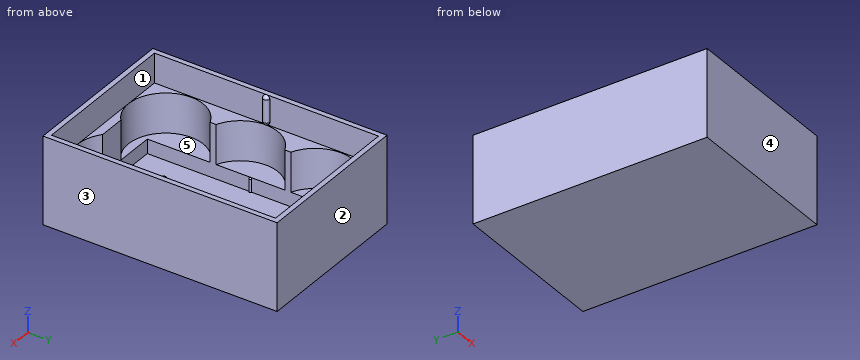
```python
from build123d import *

# Parameters (mm, degrees)
F0_W      = 94
F0_H      = 137.5
F1_DEPTH  = 2.5
F2_W      = 94
F2_H      = 137.5
F2_W_2    = 62
F2_H_2    = 123
F3_DEPTH  = 8.5
F4_W      = 94
F4_H      = 137.5
F5_DEPTH  = 23.5
F6_W      = 62
F6_H      = 123
F7_DEPTH  = 23.501
F8_W      = 94
F8_H      = 137.5
F8_W_2    = 90
F8_H_2    = 133.5
F9_DEPTH  = 17.5
F11_ANGLE = 180
F13_ANGLE = 180
F14_W     = 0.75
F14_H     = 7.75
F16_W     = 0.75
F16_H     = 7.75
F19_DEPTH = 1
F20_DEPTH = 1
F21_DEPTH = 1
F22_DEPTH = 1


with BuildPart() as f1:
    # F0 (on Top) → F1 (new body)
    with BuildSketch(Plane.XY):
        Rectangle(F0_W, F0_H)
    extrude(amount=F1_DEPTH)

    # F2 (on face) → F3 (join)
    with BuildSketch(Plane.XY.offset(2.5)):
        Rectangle(F2_W, F2_H)
        Rectangle(F2_W_2, F2_H_2, mode=Mode.SUBTRACT)
    extrude(amount=F3_DEPTH)

    # F4 (on face) → F5 (join)
    with BuildSketch(Plane.XY.offset(11)):
        Rectangle(F4_W, F4_H)
        with BuildLine():
            ThreePointArc((-22.25, 22.25), (-37.9831258814, 60.2331258814), (0, 44.5))
            ThreePointArc((0, 44.5), (22.25, 66.75), (44.5, 44.5))
            ThreePointArc((44.5, 44.5), (37.9831258872, 28.7668741244), (22.2500000164, 22.25))
            ThreePointArc((22.2500000164, 22.25), (37.9831258872, 15.7331258756), (44.5, 0))
            ThreePointArc((44.5, 0), (37.9831258814, -15.7331258814), (22.25, -22.25))
            ThreePointArc((22.25, -22.25), (37.9831258814, -28.7668741186), (44.5, -44.5))
            ThreePointArc((44.5, -44.5), (22.25, -66.75), (0, -44.5))
            ThreePointArc((0, -44.5), (-37.983125897, -60.2331258658), (-22.249999956, -22.25))
            ThreePointArc((-22.249999956, -22.25), (-44.5, -2.2e-08), (-22.25, 22.25))
        make_face(mode=Mode.SUBTRACT)
    extrude(amount=F5_DEPTH)

    # F6 (on face) → F7 (cut, through all)
    with BuildSketch(Plane.XY.offset(11)):
        Rectangle(F6_W, F6_H)
    extrude(amount=F7_DEPTH, mode=Mode.SUBTRACT)

    # F8 (on face) → F9 (join)
    with BuildSketch(Plane.XY.offset(34.5)):
        Rectangle(F8_W, F8_H)
        Rectangle(F8_W_2, F8_H_2, mode=Mode.SUBTRACT)
    extrude(amount=F9_DEPTH)

    # F10 (on face) → F11 (revolve)
    with BuildSketch(Plane.YZ.offset(-45)):
        with BuildLine():
            Line((0, 36.5), (0, 34.5))
            ThreePointArc((0, 34.5), (1.4142135624, 35.0857864376), (2, 36.5))
            Line((2, 36.5), (2, 50))
            ThreePointArc((2, 50), (1.4142135624, 51.4142135624), (0, 52))
            Line((0, 52), (0, 50))
            Line((0, 50), (0, 36.5))
        make_face()
    revolve(axis=Axis((-45, 0, 43.25), (0, 0, -1)), revolution_arc=F11_ANGLE)

    # F12 (on face) → F13 (revolve)
    with BuildSketch(Plane(origin=(45, 0, 0), x_dir=(0, -1, 0), z_dir=(-1, 0, 0))):
        with BuildLine():
            ThreePointArc((-2, 36.5), (-1.4142135624, 35.0857864376), (0, 34.5))
            Line((0, 34.5), (0, 36.5))
            Line((0, 36.5), (0, 50))
            Line((0, 50), (-2, 50))
            Line((-2, 50), (-2, 36.5))
        make_face()
        with BuildLine():
            Line((-2, 50), (0, 50))
            Line((0, 50), (0, 52))
            ThreePointArc((0, 52), (-1.4142135624, 51.4142135624), (-2, 50))
        make_face()
    revolve(axis=Axis((45, 0, 43.25), (0, 0, 1)), revolution_arc=F13_ANGLE)

    # F14 (on face) → F15 (revolve)
    with BuildSketch(Plane.YZ.offset(-31)):
        with BuildLine():
            ThreePointArc((0.75, 10.25), (0.5303300859, 10.7803300859), (0, 11))
            Line((0, 11), (0, 10.25))
            Line((0, 10.25), (0.75, 10.25))
        make_face()
        with Locations((0.375, 6.375)):
            Rectangle(F14_W, F14_H)
    revolve(axis=Axis((-31, 0, 6.75), (0, 0, -1)))

    # F16 (on face) → F17 (revolve)
    with BuildSketch(Plane(origin=(31, 0, 0), x_dir=(0, -1, 0), z_dir=(-1, 0, 0))):
        with Locations((-0.375, 6.375)):
            Rectangle(F16_W, F16_H)
        with BuildLine():
            Line((-0.75, 10.25), (0, 10.25))
            Line((0, 10.25), (0, 11))
            ThreePointArc((0, 11), (-0.5303300859, 10.7803300859), (-0.75, 10.25))
        make_face()
    revolve(axis=Axis((31, 0, 6.75), (0, 0, 1)))

    # F19 (add): a face of the model
    f19_faces = [f1.faces().sort_by_distance(p)[0] for p in [
        (47, 0, 26),
    ]]
    extrude(f19_faces, amount=F19_DEPTH)

    # F20 (add): a face of the model
    f20_faces = [f1.faces().sort_by_distance(p)[0] for p in [
        (-47, 0, 26),
    ]]
    extrude(f20_faces, amount=F20_DEPTH)

    # F21 (add): a face of the model
    f21_faces = [f1.faces().sort_by_distance(p)[0] for p in [
        (0, -68.75, 26),
    ]]
    extrude(f21_faces, amount=F21_DEPTH)

    # F22 (add): a face of the model
    f22_faces = [f1.faces().sort_by_distance(p)[0] for p in [
        (0, 68.75, 26),
    ]]
    extrude(f22_faces, amount=F22_DEPTH)


solid = f1.part
```
Source: CAD feature listing. Evaluate the final solid. Frame: model axes, mm. Face numbers are marked on the shaded views. A direction names the side the tool comes from. Round coordinates to 2 decimals unless told otherwise and drop trailing zeros. Order: outer loops, then holes, each group sorted by start corner. A loop starts at its lowest first (then second) coordinate and runs counter-clockwise, first axis right, second up. Notation, with made-up numbers: (62, 59.5) -> (108, 59.5) arc R25 cw to (108, 84.5) -> close; hole circle Ø9 at (83, -10). An arc over 180 degrees is marked (long way). One line per item, written item: value. Start each with the question number.
Q1. Access query for the marked faces 4 and 5. Directions: +Z, -Z, +X, -X, +Y, -Y. A direction counts if a zero-diameter tool reaches every point of the face in a straight line with its end or side. Return the directions, or none.
Q2. Section query C-C (x = 24). Return the cut outline in (y, z), plus the area to 3 significant figures.
Q3. Draft query along X for the marked faces 1, 2 and 3. Return one class per face: pulls with the +X half, pulls with the -X half, needs draft (parallel to the pull), parting line crosses it, or undercut.
Q4. Pin query (flat end, axial travel): pin 1 (11 mm diameter, centred on x = 36, y = 0.5, fed in from +Z); pin 2 (7 mm diameter, centred on x = -39.5, y = -10, fed in from +Z). Return the tip coordinate at first contact, or that it passes through.
Q5. Section query A-A (z = 23.5). Return the cut outline in (x, y), plus the area to 3 significant figures.
Q6. Section query D-D (z = 38.5). Return the cut outline in (x, y).
Q7. Section query B-B (y = 44.5). Return the cut outline in (x, z).
Q8. Material intervals for probe 1 along Y at (x, z) = (2, 44); probe 2 along X at (y, z) = (29.5, 36); probe 3 along Y at (x, z) = (35.5, 29.5), sorted ascending.
Findings below:
1. face 4: +Z, -Z, +X, -X, -Y
1. face 5: +Z
2. outline: (-69.75, 0) -> (69.75, 0) -> (69.75, 52) -> (66.75, 52) -> (66.75, 34.5) -> (66.68, 34.5) -> (66.68, 11) -> (61.5, 11) -> (61.5, 2.5) -> (-61.5, 2.5) -> (-61.5, 11) -> (-66.68, 11) -> (-66.68, 34.5) -> (-66.75, 34.5) -> (-66.75, 52) -> (-69.75, 52) -> close
2. area: 738 mm²
3. face 1: undercut
3. face 2: needs draft
3. face 3: pulls with the +X half
4. pin 1: z = 11
4. pin 2: z = 34.5
5. outline: (-48, -69.75) -> (48, -69.75) -> (48, 69.75) -> (-48, 69.75) -> close; hole (-31, -24.04) arc R22.25 ccw (long way) to (-7.9, -61.5) -> (7.9, -61.5) arc R22.25 ccw (long way) to (31, -24.04) -> (31, -20.46) arc R22.25 ccw to (31, 20.46) -> (31, 24.04) arc R22.25 ccw (long way) to (7.9, 61.5) -> (-7.9, 61.5) arc R22.25 ccw (long way) to (-31, 24.04) -> (-31, 20.46) arc R22.25 ccw to (-31, -20.46) -> close
5. area: 3,010 mm²
6. outline: (-48, -69.75) -> (48, -69.75) -> (48, 69.75) -> (-48, 69.75) -> close; hole (-45, -66.75) -> (45, -66.75) -> (45, -2) arc R2 cw to (45, 2) -> (45, 66.75) -> (-45, 66.75) -> (-45, 2) arc R2 cw to (-45, -2) -> close
7. outline: (-48, 0) -> (48, 0) -> (48, 52) -> (45, 52) -> (45, 34.5) -> (44.5, 34.5) -> (44.5, 11) -> (31, 11) -> (31, 2.5) -> (-31, 2.5) -> (-31, 11) -> (-44.5, 11) -> (-44.5, 34.5) -> (-45, 34.5) -> (-45, 52) -> (-48, 52) -> close
8. probe 1: -69.75 to -66.75, 66.75 to 69.75
8. probe 2: -48 to -45, 45 to 48
8. probe 3: -69.75 to -62.37, -26.63 to -17.87, 17.87 to 26.63, 62.37 to 69.75
